```python
from build123d import *

# Parameters (mm, degrees)
F2_W     = 15
F2_H     = 15
F3_DEPTH = 3
F4_W     = 3
F4_H     = 15
F5_DEPTH = 16
F6_R     = 7.49999
F8_D     = 5
F7_R     = 5
F9_DEPTH = 4


# Not quite as in the source:
# - a fillet or chamfer is up to 0.001 mm smaller than in the source, because OpenCascade refuses the exact size


with BuildPart() as f3:
    # F2 (on Top) → F3 (new body)
    with BuildSketch(Plane.XY):
        Rectangle(F2_W, F2_H)
    extrude(amount=-F3_DEPTH)

    # F4 (on face) → F5 (join)
    with BuildSketch(Plane.XY):
        with Locations((-6, 0)):
            Rectangle(F4_W, F4_H)
        Rectangle(F4_W, F4_H)
        with Locations((6, 0)):
            Rectangle(F4_W, F4_H)
    extrude(amount=F5_DEPTH)

    # F6 (radius 7.5 in the source; OpenCascade refuses exactly that, so slightly less here)
    f6_edges = [f3.edges().sort_by_distance(p)[0] for p in [
        (-6, 7.5, 16),
        (0, 7.5, 16),
        (6, 7.5, 16),
        (-6, -7.5, 16),
        (0, -7.5, 16),
        (6, -7.5, 16),
    ]]
    fillet(f6_edges, radius=F6_R)

    # F8 (through all)
    with Locations(Plane(origin=(-7.5, 0, 0), x_dir=(0, -1, 0), z_dir=(-1, 0, 0))):
        with Locations((0, 8.5)):
            Hole(F8_D / 2)

    # F7 (on face) → F9 (join)
    with BuildSketch(Plane(origin=(-7.5, 0, 0), x_dir=(0, -1, 0), z_dir=(-1, 0, 0))):
        with Locations((0, 8.5)):
            Circle(F7_R)
        Polygon((-4.6188021535, 8.5), (-2.3094010768, 12.5), (2.3094010768, 12.5), (4.6188021535, 8.5), (2.3094010768, 4.5), (-2.3094010768, 4.5), align=None, mode=Mode.SUBTRACT)
    extrude(amount=F9_DEPTH)


solid = f3.part
```
Can you work these out from the model? Positions are in its coordinate system, mm. A direction names the side the tool comes from. Round coordinates to 2 decimals unless told otherwise and drop trailing zeros. Loops run counter-clockwise (first coordinate to the right, second up) from the corner with the lowest first, then second, coordinate; pieces in that order, holes last. Notation, with made-up numbers: M 44,11 L 50,11 A12 cw 50,27 Z; hole C 4,44.25 d6. An arc over 180 degrees is marked long. Write item = value, one per line. Start each with the question number.
(1) Suppose I cut it at D-D on z = 4.25. Write out the boundary of the cut face in (x, y), plus the area to 3 significant figures.
(2) Suppose I cut it at A-A on z = 9.25. Give the number of separate pieces and of enclosed holes in the cut face, plus the area to 3 significant figures.
(3) I need wall thicknesses on line 1 along X through (y, z) = (6.5, 5.25); line 2 along Z through (x, y) = (6.95, 0); line 3 along X through (y, z) = (-3.25, 5.5). Which ranges of each line are inside material? Lowest first, please.
(4) I'm going to push flat-ended pins straight in: P1, Ø3, axis at y = 0, z = 8.5, coming from the -X side; P2, Ø2, axis at x = -10, y = 0.5, coming from the -Z side; P3, Ø0.9, axis at x = 3, y = 1, coming from the +Z side; P4, Ø1.5, axis at x = -9, y = -2.5, coming from the -Z side. Where does each tip first touch, or does it pass through?
(5) If we mould it in two halves opening along Z, with no side actions, what happens to faces 4 (the face through (0.021, 5.245, 13.861)), 5 (the face through (0, 7.5, 1)), 6 (the face through (-9, 0, 12.5))? For each: released by +Z, released by -Z, zero draft, split by the parting line, or undercut.
(6) Which directions (+Z, -Z, +X, -X, +Y, -Y) give clear straight access to the entire face, cutting with the end or side of a thin tool? Please do faces 1 (the face through (-4.5, -2, 6)), 2 (the face through (-9.472, 3.448, 6.472)), 3 (the face through (7.5, 0, 5)).
Answer block:
q1.outline = M -11.5,-2.63 L -7.5,-2.63 L -7.5,-7.5 L -4.5,-7.5 L -4.5,7.5 L -7.5,7.5 L -7.5,2.63 L -11.5,2.63 Z; M -1.5,-7.5 L 1.5,-7.5 L 1.5,7.5 L -1.5,7.5 Z; M 4.5,-7.5 L 7.5,-7.5 L 7.5,7.5 L 4.5,7.5 Z
q1.area = 156 mm²
q2.separate_pieces = 6
q2.enclosed_holes = 0
q2.area = 97.5 mm²
q3.line_1 = -7.5 to -4.5, -1.5 to 1.5, 4.5 to 7.5
q3.line_2 = -3 to 6, 11 to 16
q3.line_3 = -11.5 to -4.5, -1.5 to 1.5, 4.5 to 7.5
q4.P1 = through
q4.P2 = 3.5
q4.P3 = 0
q4.P4 = 3.82
q5.face_4 = released by +Z
q5.face_5 = zero draft
q5.face_6 = undercut
q6.face_1 = +Z, +Y, -Y
q6.face_2 = -X
q6.face_3 = +Z, -Z, +X, +Y, -Y
